Build history of the part. All positions in model axes, mm. Face numbers are marked on the shaded views. A direction names the side the tool comes from. Coordinates: 2 decimals unless noted, no trailing zeros. Order: outer loops, then holes, each group sorted by start corner. A loop starts at its lowest first (then second) coordinate and runs counter-clockwise, first axis right, second up. Notation, with made-up numbers: M 1,72 L 10,72 A36 ccw 10,111 Z; hole C 5.25,-11.75 d1. An arc over 180 degrees is marked long. Use a Markdown table: item, result. Add a question column.
from build123d import *

# Parameters (mm, degrees)
SKETCH_3_W               = 28
SKETCH_3_H               = 6
CUT_EXTRUDE_1_DEPTH      = 30
CUT_EXTRUDE_1_DEPTH_BACK = 30
FILLET_1_R               = 3


with BuildPart() as part:
    # Эскиз2 → Повернуть1 (revolve)
    with BuildSketch(Plane.XY):
        Polygon((-94, 12.5), (0, 12.5), (0, 29), (86, 18.440527762), (86, 0), (-94, 0), align=None)
    revolve(axis=Axis((0, 0, 0), (1, 0, 0)))

    # Эскиз3 → Вырез-Вытянуть1 (cut, two sides)
    with BuildSketch(Plane.XY) as cut_extrude_1_sk:
        with BuildLine():
            Line((32.5, 8.5), (55.5, 8.5))
            ThreePointArc((55.5, 8.5), (64, 0), (55.5, -8.5))
            Line((55.5, -8.5), (32.5, -8.5))
            ThreePointArc((32.5, -8.5), (24, 0), (32.5, 8.5))
        make_face()
        with Locations((-80, -9.5)):
            Rectangle(SKETCH_3_W, SKETCH_3_H)
        with Locations((-80, 9.5)):
            Rectangle(SKETCH_3_W, SKETCH_3_H)
    extrude(amount=CUT_EXTRUDE_1_DEPTH, mode=Mode.SUBTRACT)
    extrude(cut_extrude_1_sk.sketch, amount=-CUT_EXTRUDE_1_DEPTH_BACK, mode=Mode.SUBTRACT)

    # Скругление1
    fillet_1_edges = [part.edges().sort_by_distance(p)[0] for p in [
        (0, -12.5, 0),
    ]]
    fillet(fillet_1_edges, radius=FILLET_1_R)


solid = part.part
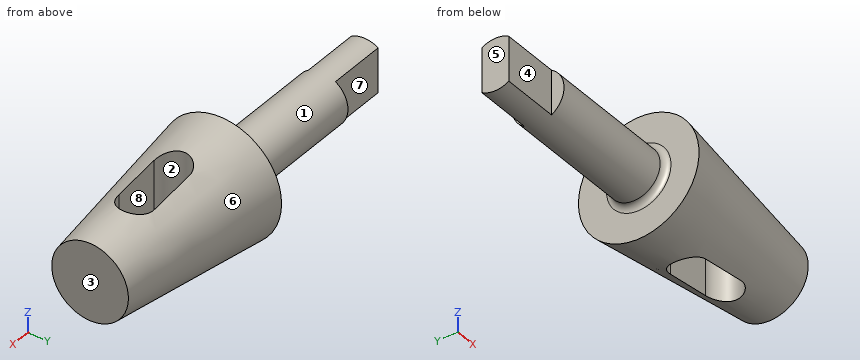
(1) Slice it at B-B on z = 0. Give the cut face in (x, y).
(2) Mould opens along X. For the marked faces 5, 6, 7 and 8 say: released by +X, released by -X, zero draft, split by the parting line, or undercut.
(3) Which spindle directions (+Z, -Z, +X, -X, +Y, -Y) get a long thin tool onto all of the face, cutting with end or side? Do the marked faces 1, 2, 3 and 4. Say none if no direction does.
(4) Drill centre lines: line 1 along X through (y, z) = (1, -13); line 2 along X through (y, z) = (0.5, 15); line 3 along Z through (x, y) = (-49, 0.5). Where is each one in solid material? Low to high. Write a range as from..to.
(5) Drop flat-ended pins along their axis: P1, Ø6.5, axis at y = -9.5, z = 4, coming from the -X side; P2, Ø10, axis at x = 6.5, y = 16, coming from the -Z side; P3, Ø1.5, axis at y = 16.5, z = -21, coming from the -X side; P4, Ø12, axis at x = -30, z = 4.5, coming from the -Y side. Give the stop position or say it passes through.
(6) Slice it at C-C on x = 71.5. Give the cut face in (y, z), and give its area (3 significant figures).
(7) Slice it at A-A on y = 0. Give the cut face in (x, z), and give its area (3 significant figures).
Solutions:
| question | item | result |
|---|---|---|
| 1 | outline | M -94,-6.5 L -66,-6.5 L -66,-12.5 L -3,-12.5 A3 cw 0,-15.5 L 0,-29 L 86,-18.44 L 86,18.44 L 0,29 L 0,15.5 A3 cw -3,12.5 L -66,12.5 L -66,6.5 L -94,6.5 Z; hole M 32.5,-8.5 L 55.5,-8.5 A8.5 ccw 55.5,8.5 L 32.5,8.5 A8.5 ccw Z |
| 2 | face 5 | released by -X |
| 2 | face 6 | released by +X |
| 2 | face 7 | zero draft |
| 2 | face 8 | undercut |
| 3 | face 1 | -X |
| 3 | face 2 | +Z, -Z |
| 3 | face 3 | +Z, -Z, +X, +Y, -Y |
| 3 | face 4 | +Z, -Z, -X, -Y |
| 4 | line 1 | -1.29..24.06, 63.94..86 |
| 4 | line 2 | -0.04..24.01, 63.99..86 |
| 4 | line 3 | -12.49..12.49 |
| 5 | P1 | x = -94 |
| 5 | P2 | z = -26.07 |
| 5 | P3 | x = 0 |
| 5 | P4 | y = -12.5 |
| 6 | outline | C 0,0 d40.44 |
| 6 | area | 1,280 mm² |
| 7 | outline | M -94,-12.5 L -3,-12.5 A3 cw 0,-15.5 L 0,-29 L 24,-26.05 L 24,26.05 L 0,29 L 0,15.5 A3 cw -3,12.5 L -94,12.5 Z; M 64,-21.14 L 86,-18.44 L 86,18.44 L 64,21.14 Z |
| 7 | area | 4,550 mm² |
